Read the model definition and answer for the solid it produces. Units are mm, in the model's axes. Face numbers are marked on the shaded views. A direction names the side the tool comes from. Round coordinates to 2 decimals unless told otherwise and drop trailing zeros. Order: outer loops, then holes, each group sorted by start corner. A loop starts at its lowest first (then second) coordinate and runs counter-clockwise, first axis right, second up. Notation, with made-up numbers: (63.25, 14) - (104.25, 14) arc R16 cw to (104.25, 31) - close; hole circle Ø8 at (70.25, -38). An arc over 180 degrees is marked (long way). Answer as a JSON object with one key per item and string values. Group by question number.
Q1. A cutting plane is placed at B-B on y = 9.7. Determine the outline of the cut face in (x, z), and give its area (3 significant figures).
Q2. Consider line 1 (Z direction, x = 2.9, y = 9.7); line 2 (X direction, y = 12, z = 0.75); line 3 (Y direction, x = 3, z = 2.5). Determine where each line is inside the solid, lowest interval first.
Q3. A tool of negligible diameter and unlimited length cuts with its end or side. For the marked faces 1 and 2, from which of +Z, -Z, +X, -X, +Y, -Y can it reach the whole face along a straight path? Write none if from no direction.
Q4. Given pin 1 Ø3.5 at (y, z) = (10, 4) entering from -X, flat-ended and moving along its own axis, determine where the tip first touches the part or whether it passes through.
Q5. The mould has two halves that part along Z. Classify the marked faces 3, 4, 5 and 6: pulls with the +Z half, pulls with the -Z half, needs draft (parallel to the pull), parting line crosses it, or undercut.
Q6. A cutting plane is placed at A-A on z = 3.3. Determine the outline of the cut face in (x, y).
Q7. A cutting plane is placed at C-C on x = 0. Determine the outline of the cut face in (y, z).
```python
from build123d import *

# Parameters (mm, degrees)
SKETCH_1_R          = 3.85
EXTRUDE_1_DEPTH     = 6.6
EXTRUDE_START       = -6.6
EXTRUDE_2_DEPTH     = 6.6
SKETCH_3_R          = 2.5
EXTRUDE_3_DEPTH     = 2.5
FILLET_1_R          = 1
SKETCH_4_R          = 1.65
CUT_EXTRUDE_1_DEPTH = 10.6
FILLET_2_R          = 1


with BuildPart() as part:
    # 草图1 → 凸台-拉伸1 (new body)
    with BuildSketch(Plane.XY):
        Circle(SKETCH_1_R)
    extrude(amount=EXTRUDE_1_DEPTH)

    # 草图2 → 凸台-拉伸2 (add)
    with BuildSketch(Plane.XY.offset(6.6).offset(EXTRUDE_START)):
        with BuildLine():
            Line((3.85, 0), (3.85, 14.5))
            Line((3.85, 14.5), (2.35, 14.5))
            Line((2.35, 14.5), (2.35, 3.049590136))
            ThreePointArc((2.35, 3.049590136), (3.454706934, 1.699264547), (3.85, 0))
        make_face()
    extrude(amount=EXTRUDE_2_DEPTH)

    # 草图3 → 凸台-拉伸3 (add)
    with BuildSketch(Plane.XY.offset(6.6)):
        Circle(SKETCH_3_R)
    extrude(amount=EXTRUDE_3_DEPTH)

    # 圆角1
    fillet_1_edges = [part.edges().sort_by_distance(p)[0] for p in [
        (-2.5, 0, 6.6),
        (-2.5, 0, 9.1),
    ]]
    fillet(fillet_1_edges, radius=FILLET_1_R)

    # 草图4 → 切除-拉伸1 (cut)
    with BuildSketch(Plane.ZY.offset(-2.35)):
        with Locations(Location((3.3, 9.7, 0), (0, 0, 270))):
            Circle(SKETCH_4_R)
    extrude(amount=-CUT_EXTRUDE_1_DEPTH, mode=Mode.SUBTRACT)

    # 圆角2
    fillet_2_edges = [part.edges().sort_by_distance(p)[0] for p in [
        (3.1, 14.5, 6.6),
        (3.1, 14.5, 0),
    ]]
    fillet(fillet_2_edges, radius=FILLET_2_R)


solid = part.part
```
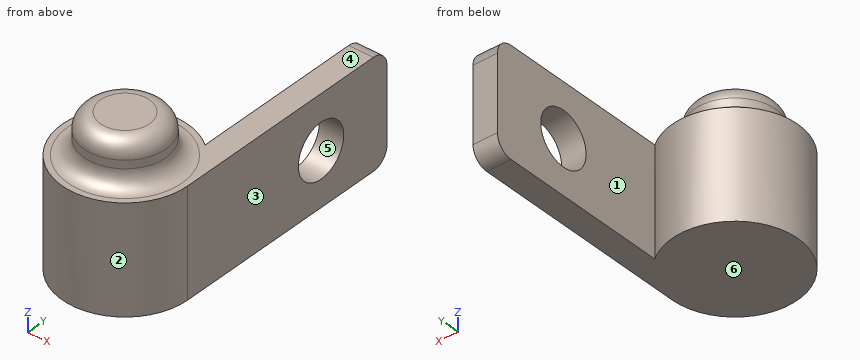
Result set:
{
 "1": {"outline": "(2.35, 0) - (3.85, 0) - (3.85, 1.65) - (2.35, 1.65) - close; (2.35, 4.95) - (3.85, 4.95) - (3.85, 6.6) - (2.35, 6.6) - close", "area": "4.95 mm²"},
 "2": {"line 1": "z = 0 to 1.65, 4.95 to 6.6", "line 2": "x = 2.35 to 3.85", "line 3": "y = -2.41 to 8.26, 11.14 to 14.5"},
 "3": {"face 1": "+Z, -Z, +Y", "face 2": "+Z, -Z"},
 "4": {"pin 1": "stops at x = 2.35"},
 "5": {"face 3": "needs draft", "face 4": "pulls with the +Z half", "face 5": "undercut", "face 6": "pulls with the -Z half"},
 "6": {"outline": "(2.35, 3.05) arc R3.85 ccw (long way) to (3.85, 0) - (3.85, 8.05) - (2.35, 8.05) - close; (2.35, 11.35) - (3.85, 11.35) - (3.85, 14.5) - (2.35, 14.5) - close"},
 "7": {"outline": "(-3.85, 0) - (3.85, 0) - (3.85, 6.6) - (3.5, 6.6) arc R1 cw to (2.5, 7.6) - (2.5, 8.1) arc R1 ccw to (1.5, 9.1) - (-1.5, 9.1) arc R1 ccw to (-2.5, 8.1) - (-2.5, 7.6) arc R1 cw to (-3.5, 6.6) - (-3.85, 6.6) - close"}
}
